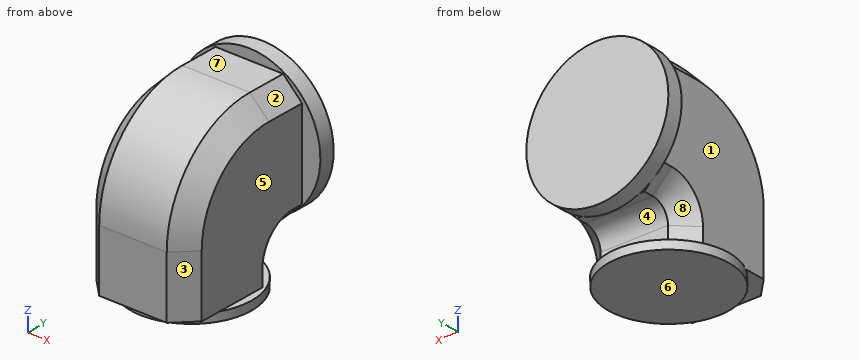
```python
from build123d import *

# Parameters (mm, degrees)
SKETCH1_R      = 4.427139884
EXTRUDE1_DEPTH = 0.644658235
EXTRUDE2_DEPTH = 3.885892792
SKETCH3_R      = 5.238234522
EXTRUDE3_DEPTH = 1.161266807
CHAMFER1_SIZE  = 1.397


with BuildPart() as part:
    # Sketch1 → Extrude1 (new body)
    with BuildSketch(Plane.XY):
        with Locations((0, 20.585351579)):
            Circle(SKETCH1_R)
    extrude(amount=EXTRUDE1_DEPTH)

    # Sketch2 → Extrude2 (add, symmetric)
    with BuildSketch(Plane(origin=(0, 0, 0), x_dir=(0, 0, -1), z_dir=(1, 0, 0))):
        with BuildLine():
            Line((-0.644658235, 15.505020105), (-0.644658235, 23.59311727))
            Line((-0.644658235, 23.59311727), (-1.832887116, 23.59311727))
            ThreePointArc((-1.832887116, 23.59311727), (-2.764654054, 23.979067772), (-3.150604557, 24.910834711))
            Line((-3.150604557, 24.910834711), (-3.150604557, 25.650777017))
            Line((-3.150604557, 25.650777017), (-12.398423576, 25.650777017))
            Line((-12.398423576, 25.650777017), (-12.398423576, 22.749820493))
            ThreePointArc((-12.398423576, 22.749820493), (-10.27647067, 17.62697301), (-5.153623188, 15.505020105))
            Line((-5.153623188, 15.505020105), (-0.644658235, 15.505020105))
        make_face()
    extrude(amount=EXTRUDE2_DEPTH, both=True)

    # Sketch3 → Extrude3 (add)
    with BuildSketch(Plane(origin=(0, 25.650777017, 0), x_dir=(1, 0, 0), z_dir=(0, 1, 0))):
        with Locations(Location((0, -7.934882504, 0), (0, 0, 65.970774096))):
            Circle(SKETCH3_R)
    extrude(amount=EXTRUDE3_DEPTH)

    # Chamfer1
    # the kernel refuses this chamfer: 1.397 mm, written as the material it takes off along each edge
    with BuildSketch(Plane(origin=(-3.885892792, 24.910834711, 1.832887116), x_dir=(0, -1, 0), z_dir=(0, 0, -1))) as chamfer1_piece_1:
        Polygon((1.317717441 + CHAMFER1_SIZE, 0), (1.317717441, -CHAMFER1_SIZE), (1.317717441, 0), align=None)
    revolve(axis=Axis((-3.885892792, 24.910834711, 1.832887116), (-1, 0, 0)), revolution_arc=90, mode=Mode.SUBTRACT)
    with BuildSketch(Plane(origin=(-3.885892792, 24.910834711, 3.150604557), x_dir=(-0.027495876610586344, 0, 0.9996219169112966), z_dir=(0, 1, 0))) as chamfer1_piece_2:
        Polygon((CHAMFER1_SIZE * 0.999621916911, CHAMFER1_SIZE * 0.0274958766106), (-CHAMFER1_SIZE * 0.0274958766106, CHAMFER1_SIZE * 0.999621916911), (0, 0), align=None)
    extrude(amount=0.739942306, mode=Mode.SUBTRACT)
    with BuildSketch(Plane(origin=(-3.885892792, 25.650777017, 12.398423576), x_dir=(-0.027495876610586365, 0, -0.9996219169112968), z_dir=(0, -1, 0))) as chamfer1_piece_3:
        Polygon((CHAMFER1_SIZE * 0.999621916911, CHAMFER1_SIZE * 0.0274958766106), (-CHAMFER1_SIZE * 0.0274958766106, CHAMFER1_SIZE * 0.999621916911), (0, 0), align=None)
    extrude(amount=2.900956524, mode=Mode.SUBTRACT)
    with BuildSketch(Plane(origin=(-3.885892792, 22.749820493, 5.153623188), x_dir=(0, 0, 1), z_dir=(0, 1, 0))) as chamfer1_piece_4:
        Polygon((7.244800387 - CHAMFER1_SIZE, 0), (7.244800387, CHAMFER1_SIZE), (7.244800387, 0), align=None)
    revolve(axis=Axis((-3.885892792, 22.749820493, 5.153623188), (1, 0, 0)), revolution_arc=90, mode=Mode.SUBTRACT)
    with BuildSketch(Plane(origin=(3.885892792, 15.505020105, 5.153623188), x_dir=(0.027495876610586393, 0.9996219169112966, 0), z_dir=(0, 0, -1)), Plane(origin=(-3.885892792, 15.505020105, 5.153623188), x_dir=(0.9996219169112968, -0.027495876610586046, 0), z_dir=(0, 0, -1))) as chamfer1_piece_5:
        Polygon((CHAMFER1_SIZE * 0.999621916911, -CHAMFER1_SIZE * 0.0274958766106), (-CHAMFER1_SIZE * 0.0274958766106, -CHAMFER1_SIZE * 0.999621916911), (0, 0), align=None)
    extrude(amount=8.101606087, mode=Mode.SUBTRACT)
    with BuildSketch(Plane(origin=(3.885892792, 23.59311727, 0.644658235), x_dir=(0.027495876610586393, -0.9996219169112966, 0), z_dir=(0, 0, 1))) as chamfer1_piece_6:
        Polygon((CHAMFER1_SIZE * 0.999621916911, -CHAMFER1_SIZE * 0.0274958766106), (-CHAMFER1_SIZE * 0.0274958766106, -CHAMFER1_SIZE * 0.999621916911), (0, 0), align=None)
    extrude(amount=1.188228881, mode=Mode.SUBTRACT)
    with BuildSketch(Plane(origin=(3.885892792, 24.910834711, 1.832887116), x_dir=(0, -1, 0), z_dir=(0, 0, -1))) as chamfer1_piece_7:
        Polygon((1.317717441 + CHAMFER1_SIZE, 0), (1.317717441, CHAMFER1_SIZE), (1.317717441, 0), align=None)
    revolve(axis=Axis((3.885892792, 24.910834711, 1.832887116), (-1, 0, 0)), revolution_arc=90, mode=Mode.SUBTRACT)
    with BuildSketch(Plane(origin=(3.885892792, 24.910834711, 3.150604557), x_dir=(0.027495876610586344, 0, 0.9996219169112966), z_dir=(0, 1, 0))) as chamfer1_piece_8:
        Polygon((CHAMFER1_SIZE * 0.999621916911, -CHAMFER1_SIZE * 0.0274958766106), (-CHAMFER1_SIZE * 0.0274958766106, -CHAMFER1_SIZE * 0.999621916911), (0, 0), align=None)
    extrude(amount=0.739942306, mode=Mode.SUBTRACT)
    with BuildSketch(Plane(origin=(3.885892792, 25.650777017, 12.398423576), x_dir=(0.027495876610586365, 0, -0.9996219169112968), z_dir=(0, -1, 0))) as chamfer1_piece_9:
        Polygon((CHAMFER1_SIZE * 0.999621916911, -CHAMFER1_SIZE * 0.0274958766106), (-CHAMFER1_SIZE * 0.0274958766106, -CHAMFER1_SIZE * 0.999621916911), (0, 0), align=None)
    extrude(amount=2.900956524, mode=Mode.SUBTRACT)
    with BuildSketch(Plane(origin=(3.885892792, 22.749820493, 5.153623188), x_dir=(0, 0, 1), z_dir=(0, 1, 0))) as chamfer1_piece_10:
        Polygon((7.244800387 - CHAMFER1_SIZE, 0), (7.244800387, -CHAMFER1_SIZE), (7.244800387, 0), align=None)
    revolve(axis=Axis((3.885892792, 22.749820493, 5.153623188), (1, 0, 0)), revolution_arc=90, mode=Mode.SUBTRACT)
    with BuildSketch(Plane(origin=(-3.885892792, 23.59311727, 0.644658235), x_dir=(-0.027495876610586393, -0.9996219169112966, 0), z_dir=(0, 0, 1))) as chamfer1_piece_11:
        Polygon((CHAMFER1_SIZE * 0.999621916911, CHAMFER1_SIZE * 0.0274958766106), (-CHAMFER1_SIZE * 0.0274958766106, CHAMFER1_SIZE * 0.999621916911), (0, 0), align=None)
    extrude(amount=1.188228881, mode=Mode.SUBTRACT)


solid = part.part
```
Part model, mm, in its own coordinate system. Face numbers are marked on the shaded views. A direction names the side the tool comes from. Coordinates: 2 decimals unless noted, no trailing zeros. Loops run counter-clockwise (first coordinate to the right, second up) from the corner with the lowest first, then second, coordinate; pieces in that order, holes last. Notation, with made-up numbers: (21, 62.5) - (38, 62.5) arc R9 cw to (38, 72.5) - close; hole circle Ø7 at (37, 82.5). An arc over 180 degrees is marked (long way). Write item = value, one per line. Start each with the question number.
Item 1: Cut at D-D, the plane x = -2.75. Give the cut face in (y, z).
Item 2: Cut at A-A, the plane x = 4.25. Give the cut face in (y, z), and give its area (3 significant figures).
Item 3: 3-axis set-ups, long thin cutter, end or side, ignore diameter. For the marked faces 1, 2, 3 and 4: which of +Z, -Z, +X, -X, +Y, -Y reach the whole face in a straight line?
Item 4: Wall check: L1, parallel to Z at x = 1.5, y = 22.5; L2, parallel to Y at x = -4.5, z = 7; L3, parallel to X at y = 21, z = 1.25. Give the ranges that are in metal, low to high. Write a range as from..to.
Item 5: Mould opens along Z. For the marked faces 5, 6, 7 and 8 say: released by +Z, released by -Z, zero draft, split by the parting line, or undercut.
Item 6: Cut at B-B, the plane y = 25.25. Give the cut face in (x, z).
Item 7: Cut at C-C, the plane x = 0. Give the cut face in (y, z), and give its area (3 significant figures).
Item 8: Flat gauge pins, fed straight in: pin 1 Ø2 at (x, y) = (2, 22.5) entering from +Z; pin 2 Ø1.3 at (x, z) = (-1, 1) entering from +Y; pin 3 Ø2.5 at (y, z) = (19.5, 6) entering from -X. Where does each tip first touch, or does it go through?
The answers:
q1.outline = (15.77, 0.64) - (17.12, 0.64) - (17.12, 0) - (24.05, 0) - (24.05, 0.64) - (23.33, 0.64) - (23.33, 1.83) arc R1.58 cw to (24.91, 3.41) - (25.65, 3.41) - (25.65, 3.48) - (26.81, 3.48) - (26.81, 12.39) - (25.65, 12.39) - (25.65, 12.14) - (22.75, 12.14) arc R6.98 ccw to (15.77, 5.15) - close
q2.outline = (19.35, 0) - (21.83, 0) - (21.83, 0.64) - (19.35, 0.64) - close; (25.65, 4.87) - (26.81, 4.87) - (26.81, 11) - (25.65, 11) - close
q2.area = 8.71 mm2
q3.face_1 = +Z, -X, -Y
q3.face_2 = +Z, +X, -Y
q3.face_3 = +Z, -Z, +X, -Y
q3.face_4 = +X, -X
q4.L1 = 0..12.39
q4.L2 = 25.65..26.81
q4.L3 = -3.89..3.89
q5.face_5 = zero draft
q5.face_6 = released by -Z
q5.face_7 = released by +Z
q5.face_8 = undercut
q6.outline = (-3.89, 4.55) - (-2.49, 3.15) - (2.49, 3.15) - (3.89, 4.55) - (3.89, 11) - (2.49, 12.4) - (-2.49, 12.4) - (-3.89, 11) - close
q7.outline = (15.51, 0.64) - (16.16, 0.64) - (16.16, 0) - (25.01, 0) - (25.01, 0.64) - (23.59, 0.64) - (23.59, 1.83) arc R1.32 cw to (24.91, 3.15) - (25.65, 3.15) - (25.65, 2.7) - (26.81, 2.7) - (26.81, 13.17) - (25.65, 13.17) - (25.65, 12.4) - (22.75, 12.4) arc R7.24 ccw to (15.51, 5.15) - close
q7.area = 121 mm2
q8.pin_1 = 12.4
q8.pin_2 = 24.99
q8.pin_3 = -3.89
